Could you check a few things on this model? Use its own coordinates, in mm. Face numbers are marked on the shaded views. A direction names the side the tool comes from. Coordinates: 2 decimals unless noted, no trailing zeros. Loops run counter-clockwise (first coordinate to the right, second up) from the corner with the lowest first, then second, coordinate; pieces in that order, holes last. Notation, with made-up numbers: (59.25, 27.5) -> (95.25, 27.5) arc R20 cw to (95.25, 45.5) -> close; hole circle Ø4 at (34, 49). An arc over 180 degrees is marked (long way). One line per question, with ' | ' between items.
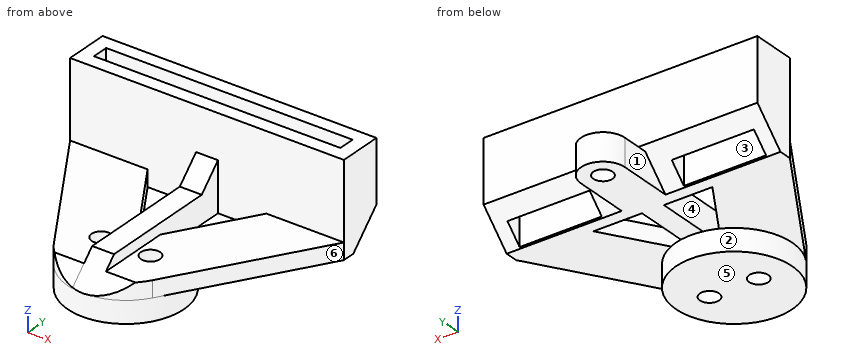
Autodesk Inventor part; units mm, degrees
ref_plane "YZ Plane" through (0, 0, 0) normal (1, 0, 0) x (0, 1, 0)
ref_plane "XZ Plane" through (0, 0, 0) normal (0, 1, 0) x (-1, 0, 0)
ref_plane "XY Plane" through (0, 0, 0) normal (0, 0, 1) x (1, 0, 0)
sketch "Sketch1" plane through (0, 0, 0) normal (0, 0, 1) x (1, 0, 0)
  circle A0 centre (4.5, 0) radius 2.2
  circle A1 centre (-4.5, 0) radius 2.2
  circle A2 centre (0, 0) radius 10.6
  circle A3 centre (4.5, 0) radius 1.75
  circle A4 centre (-4.5, 0) radius 1.75
  point P0 (0, 0)
  dimension "d0" = 3.5
  dimension "d1" = 3.5
extrude "Extrusion1" add sketch "Sketch1" along normal blind 4 contours A0 | A1 | A2
sketch "Sketch2" plane through (0, 0, 0) normal (1, 0, 0) x (0, 1, 0)
  line L0 (10.6, 4) -> (-10.6, 4)
  line L1 (-10.6, 4) -> (-5.6, 9)
  line L2 (-5.6, 9) -> (16, 9)
  line L3 (16, 9) -> (20, 13)
  line L4 (20, 13) -> (20, 21)
  line L5 (20, 21) -> (28, 21)
  line L6 (28, 21) -> (28, 4)
  line L7 (28, 4) -> (10.6, 4)
  line L8 (28, 9.6863) -> (22.3137, 4)
  line L9 (28, 9.6863) -> (36.0416, 9.6863) construction
  point P0 (0, 0)
  point P1 (0, 4)
  dimension "d4" = 135
  dimension "d5" = 5
  dimension "d6" = 45
  dimension "d7" = 8
  dimension "d8" = 8
  dimension "d9" = 4
  dimension "d10" = 8
  dimension "d11" = 20
extrude "Extrusion2" add sketch "Sketch2" along normal mid plane 4 contours L0 L1 L2 L3 L4 L5 L6 L8 L7
sketch "Sketch3" plane through (2, -10.6, 4) normal (0, 0, -1) x (-1, 0, 0)
  circle A0 centre (2, 10.6) radius 10.6
  line L0 (4, 0) -> (2, 0)
  line L1 (2, 0) -> (0, 0)
  line L2 (0, 5) -> (0, 0)
  line L3 (4, 5) -> (0, 5)
  line L4 (4, 0) -> (4, 5)
  point P0 (2, 10.6)
  point P1 (0, 0.1904)
  point P2 (4, 0.1904)
extrude "Extrusion3" cut sketch "Sketch3" against normal through all contours A0 L1 L2 | L4 L0 A0
sketch "Sketch4" plane through (-2, 20, 21) normal (0, 0, 1) x (1, 0, 0)
  line L0 (4, 0) -> (0, 0)
  line L1 (4, 8) -> (4, 0) construction
  line L2 (0, 8) -> (4, 8)
  line L3 (0, 0) -> (0, 8) construction
  line L4 (0, 8) -> (4, 8)
  line L5 (2, 8) -> (2, 0)
  line L6 (0, 0) -> (4, 0)
  line L7 (-23, 8) -> (27, 8)
  line L8 (27, 8) -> (27, 0)
  line L9 (27, 0) -> (-23, 0)
  line L10 (-23, 0) -> (-23, 8)
  line L11 (-23, 8) -> (27, 0) construction
  line L12 (27, 8) -> (-23, 0) construction
  point P0 (2, -20)
  point P1 (2, 4)
  dimension "d16" = 50
extrude "Extrusion4" add sketch "Sketch4" against normal up to surface surface through (0, 22.3137, 4) normal (0, 0.7071, -0.7071)
sketch "Sketch5" plane through (25, 20, 21) normal (1, 0, 0) x (0, 0, -1)
  line L0 (17, -9.5904) -> (17, 0)
  line L1 (19.3137, 0) -> (11.3137, 8)
  line L2 (0, 8) -> (11.3137, 8)
  line L3 (0, 0) -> (0, 8)
  line L4 (0, 0) -> (19.3137, 0)
  line L5 (17, 0) -> (17, 2.3137)
  line L6 (11.3137, 8) -> (19.3137, 0)
  point P0 (21, -20)
extrude "Extrusion5" cut sketch "Sketch5" against normal through all contours L4 L5 L1
sketch "Sketch6" plane through (25, 20, 21) normal (0, 0, 1) x (1, 0, 0)
  line L0 (0, 0) -> (-50, 0)
  line L1 (0, 0) -> (0, 8)
  line L2 (-50, 8) -> (0, 8)
  line L3 (-50, 8) -> (-50, 0)
  line L4 (0, 0) -> (0, 8)
  line L5 (0, 4) -> (-50, 4) construction
  line L6 (-50, 8) -> (-50, 0)
  line L7 (-50, 8) -> (0, 8)
  line L8 (-25, 8) -> (-25, 0) construction
  line L9 (-27, 0) -> (-23, 0)
  line L10 (-17.5, 5.5) -> (-2.5, 5.5)
  line L11 (-2.5, 5.5) -> (-2.5, 2.5)
  line L12 (-2.5, 2.5) -> (-17.5, 2.5)
  line L13 (-17.5, 2.5) -> (-17.5, 5.5)
  line L14 (-17.5, 5.5) -> (-2.5, 2.5) construction
  line L15 (-2.5, 5.5) -> (-17.5, 2.5) construction
  line L16 (-32.5, 5.5) -> (-47.5, 5.5)
  line L17 (-47.5, 5.5) -> (-47.5, 2.5)
  line L18 (-47.5, 2.5) -> (-32.5, 2.5)
  line L19 (-32.5, 2.5) -> (-32.5, 5.5)
  point P0 (-25, -20)
  point P1 (-10, 4)
  dimension "d21" = 15
  dimension "d22" = 3
  dimension "d23" = 2.5
extrude "Extrusion6" cut sketch "Sketch6" against normal through all contours L10 L11 L12 L13 | L19 L18 L17 L16
sketch "Sketch7" plane through (25, 20, 21) normal (0, 0, 1) x (1, 0, 0)
  line L0 (-17.5, 2.5) -> (-17.5, 5.5)
  line L1 (-32.5, 5.5) -> (-32.5, 2.5)
  line L2 (-17.5, 5.5) -> (-32.5, 5.5)
  line L3 (-32.5, 5.5) -> (-32.5, 2.5)
  line L4 (-32.5, 2.5) -> (-17.5, 2.5)
  line L5 (-17.5, 2.5) -> (-17.5, 5.5)
  point P0 (-25, -20)
extrude "Extrusion7" cut sketch "Sketch7" against normal blind 6
sketch "Sketch8" plane through (0, 0, 4) normal (0, 0, 1) x (1, 0, 0)
  circle A0 centre (4.5, 0) radius 1.75
  line L0 (2, 10.4096) -> (2, -10.4096)
  line L1 (2, 20) -> (25, 20)
  line L2 (25, 20) -> (8.9888, -5.618)
  arc A1 (2, -10.4096) -> (2, 10.4096) centre (0, 0) ccw
  line L3 (2, 5.8415) -> (10.849, 20)
  arc A2 (-2, -10.4096) -> (2, -10.4096) centre (0, 0) ccw
  line L4 (0, -10.6) -> (0, 30.6147)
  line L5 (-25, 20) -> (-8.9888, -5.618)
  line L6 (-2, 5.8415) -> (-10.849, 20)
  arc A3 (-2, 10.4096) -> (-2, -10.4096) centre (0, 0) ccw
  line L7 (-13.7579, -10.035) -> (-3.7579, -10.035)
  line L8 (-25, 20) -> (-2, 20)
  point P0 (0, 0)
  dimension "d29" = 12
extrude "Extrusion8" add sketch "Sketch8" along normal blind 3 contours L3 A1 L0 | L3 L1 L2 A1 picked at (5.0326, 4.687)
sketch "Sketch9" plane through (2, -10.4096, 7) normal (-1, 0, 0) x (0, 0, 1)
  line L0 (0, 2.8096) -> (-2.8096, 0)
  line L1 (-2.8096, 0) -> (0, 0)
  line L2 (0, 2.8096) -> (0, 0)
  point P0 (-7, 10.4096)
extrude "Extrusion9" cut sketch "Sketch9" against normal through all
mirror "Mirror1" about plane through (0, 0, 0) normal (1, 0, 0) of "Extrusion8", "Extrusion9"
sketch "Sketch10" plane through (0, 0, 4) normal (0, 0, -1) x (-1, 0, 0)
  circle A0 centre (0, 32.3137) radius 1.75
  circle A1 centre (0, 32.3137) radius 4
  line L0 (-4, 32.3137) -> (-4, 22.3137)
  line L1 (-25, 22.3137) -> (25, 22.3137)
  line L2 (0, 22.3137) -> (0, 32.3137) construction
  line L3 (4, 32.3137) -> (4, 22.3137)
  point P0 (0, 0)
  dimension "d36" = 8
  dimension "d34" = 3.5
  dimension "d35" = 10
extrude "Extrusion10" add sketch "Sketch10" against normal blind 5
properties part number "Lazercutlink"
Q1. We'd pull the mould along X, two halves only. Please class the marked faces 4, 5 and 6: released by +X, released by -X, zero draft, split by the parting line, or undercut.
Values follow:
face 4: undercut | face 5: zero draft | face 6: released by +X
Q2. For the marked faces 1, 2 and 3, which set-ups out of +Z, -Z, +X, -X, +Y, -Y let a thin tool reach every point of the face, with its end or its side?
Values follow:
face 1: -Z, -X, +Y | face 2: -Z | face 3: +Z
Q3. Imagine slicing it at C-C on z = 11. Write out the boundary of the cut face in (x, y).
Values follow:
outline: (-25, 20) -> (-2, 20) -> (-2, 18) -> (2, 18) -> (2, 20) -> (25, 20) -> (25, 28) -> (-25, 28) -> close; hole (-22.5, 22.5) -> (-7.5, 22.5) -> (-7.5, 25.5) -> (-22.5, 25.5) -> close; hole (7.5, 22.5) -> (22.5, 22.5) -> (22.5, 25.5) -> (7.5, 25.5) -> close
Q4. Please list where these lines run through material, in increasing order: L1, parallel to Y at x = -20, z = 18; L2, parallel to Y at x = 4.5, z = 5.5; L3, parallel to Y at x = -5, z = 5.25. Write a range as [from, to].
Values follow:
L1: y = [20, 22.5], [25.5, 28] | L2: y = [-9.1, -1.75], [1.75, 9.84], [20, 23.81] | L3: y = [-9.35, -1.68], [1.68, 10.64], [20, 23.56]
Q5. Imagine slicing it at D-D on x = 17.5. Write out the boundary of the cut face in (y, z), plus the area to 3 significant figures.
Values follow:
outline: (8, 4) -> (22.31, 4) -> (22.5, 4.19) -> (22.5, 21) -> (20, 21) -> (20, 7) -> (8, 7) -> close; (25.5, 7.19) -> (28, 9.69) -> (28, 21) -> (25.5, 21) -> close | area: 110 mm2
Q6. Imagine slicing it at B-B on y = 0. Write out the boundary of the cut face in (x, z).
Values follow:
outline: (-12.5, 4) -> (-10.6, 4) -> (-10.6, 0) -> (-6.25, 0) -> (-6.25, 7) -> (-12.5, 7) -> close; (-2.75, 0) -> (2.75, 0) -> (2.75, 7) -> (2, 7) -> (2, 9) -> (-2, 9) -> (-2, 7) -> (-2.75, 7) -> close; (6.25, 0) -> (10.6, 0) -> (10.6, 4) -> (12.5, 4) -> (12.5, 7) -> (6.25, 7) -> close
Q7. Imagine slicing it at A-A on x = 0. Write out the boundary of the cut face in (y, z).
Values follow:
outline: (-10.6, 0) -> (10.6, 0) -> (10.6, 4) -> (30.56, 4) -> (30.56, 9) -> (27.31, 9) -> (28, 9.69) -> (28, 21) -> (25.5, 21) -> (25.5, 15) -> (22.5, 15) -> (22.5, 21) -> (20, 21) -> (20, 13) -> (16, 9) -> (-5.6, 9) -> (-10.6, 4) -> close; (34.06, 4) -> (36.31, 4) -> (36.31, 9) -> (34.06, 9) -> close
Q8. For pin 1 (5.5 mm diameter, centred on x = 4.5, y = 0, fed in from +Z); pin 2 (1 mm diameter, centred on x = 18, z = 8, fed in from -Y); pin 3 (4.5 mm diameter, centred on y = -0.5, z = 7.5, fed in from -X); pin 4 (3 mm diameter, centred on x = -4.5, y = 0, fed in from -Z), each with a flat end and sliding along its axis, tell me the tip position at first contact or that it passes through.
Values follow:
pin 1: stops at z = 9 | pin 2: stops at y = 20 | pin 3: stops at x = -13.56 | pin 4: passes through
